CAD build for the part. Positions are in the model's coordinates, mm. A direction names the side the tool comes from. Coordinates: 2 decimals unless noted, no trailing zeros. Loops run counter-clockwise (first coordinate to the right, second up) from the corner with the lowest first, then second, coordinate; pieces in that order, holes last. Notation, with made-up numbers: (82, 8) -> (114, 8) arc R19 ccw to (114, 44) -> close; hole circle Ø1 at (75, 50). An arc over 180 degrees is marked (long way). Write each question's results on one line, items separated by ' | '.
Autodesk Inventor part; units mm, degrees
ref_plane "YZ Plane" through (0, 0, 0) normal (1, 0, 0) x (0, 1, 0)
ref_plane "XZ Plane" through (0, 0, 0) normal (0, 1, 0) x (-1, 0, 0)
ref_plane "XY Plane" through (0, 0, 0) normal (0, 0, 1) x (1, 0, 0)
sketch "Sketch1" plane through (0, 0, 0) normal (0, 1, 0) x (-1, 0, 0)
  line L0 (0.8453, 25) -> (0.8453, 15)
  line L1 (0.8453, 15) -> (4.8453, 15)
  line L2 (4.8453, 15) -> (4.8453, 2)
  line L3 (0.8453, 25) -> (25.8453, 25)
  line L4 (25.8453, 25) -> (25.8453, 6)
  line L5 (4.8453, 2) -> (11.8453, 2)
  line L6 (11.8453, 2) -> (14.1547, 6)
  line L7 (14.1547, 6) -> (25.8453, 6)
  point P0 (0, 0)
  dimension "d1" = 10
  dimension "d2" = 4
  dimension "d3" = 13
  dimension "d13" = 25
  dimension "d14" = 19
  dimension "d16" = 7
  dimension "d17" = 60
  dimension "d19" = 4
revolve "Revolution1" add sketch "Sketch1" angle 360 about axis through (-0.8453, 0, 25) along (-1, 0, 0)
sketch "Sketch2" plane through (-25.8453, 0, 25) normal (-1, 0, 0) x (0, 0, 1)
  circle A0 centre (0, 0) radius 13
  point P0 (-25, 0)
  dimension "d21" = 26
extrude "Extrusion1" cut sketch "Sketch2" against normal blind 15
thread "Thread1"
properties part number "00.32.012 \"Valve\"" material "Steel"
1) Two-plate mould, pull along Y, no slides. Class faces 4 (the flat face through (-10.845, 0, 25)), 5 (the cylindrical face through (-8.394, -22.804, 27.994)), 6 (the flat face through (-25.845, 12.4, 29.5)): pulls with the +Y half, pulls with the -Y half, needs draft (parallel to the pull), parting line crosses it, or undercut.
Outcome:
face 4: undercut | face 5: parting line crosses it | face 6: needs draft
2) Slice it at D-D (x = -8.25). Write the cut outline in (y, z).
Outcome:
outline: circle Ø46 at (0, 25)
3) Drill centre lines: L1, parallel to Y at x = -17.5, z = 25; L2, parallel to X at y = -16.5, z = 28.5; L3, parallel to Z at x = -20.75, y = 8.5. Where is each one in solid material? Low to high. Write a range as from..to.
Outcome:
L1: y = -19..-13, 13..19 | L2: x = -25.85..-4.85 | L3: z = 8.01..15.16, 34.84..41.99
4) Slice it at C-C (x = -20.75). Write the cut outline in (y, z), then the cut area to 3 significant figures.
Outcome:
outline: circle Ø38 at (0, 25); hole circle Ø26 at (0, 25) | area: 603 mm^2
5) Which spindle directions (+Z, -Z, +X, -X, +Y, -Y) get a long thin tool onto all of the face, cutting with end or side? Do faces 1 (the flat face through (-4.845, 5, 15)), 2 (the flat face through (-0.845, 0, 25)), 3 (the cylindrical face through (-18.5, 3.9, 37.4)). Say none if no direction does.
Outcome:
face 1: +X | face 2: +Z, -Z, +X, +Y, -Y | face 3: -X
6) Pin check, flat tips, straight feed: pin 1 (1 mm diameter, centred on y = -17.5, z = 36, fed in from -X); pin 2 (1.5 mm diameter, centred on x = -8.5, y = -18, fed in from +Z); pin 3 (8 mm diameter, centred on y = 13, z = 34, fed in from +X). Stop position of each tip, or through.
Outcome:
pin 1: stops at x = -13.48 | pin 2: stops at z = 40.21 | pin 3: stops at x = -4.85
7) Slice it at A-A (z = 25). Write the cut outline in (x, y), then the cut area to 3 significant figures.
Outcome:
outline: (-25.85, -19) -> (-14.15, -19) -> (-11.85, -23) -> (-4.85, -23) -> (-4.85, -10) -> (-0.85, -10) -> (-0.85, 10) -> (-4.85, 10) -> (-4.85, 23) -> (-11.85, 23) -> (-14.15, 19) -> (-25.85, 19) -> (-25.85, 13) -> (-10.85, 13) -> (-10.85, -13) -> (-25.85, -13) -> close | area: 553 mm^2
8) Slice it at B-B (y = 0). Write the cut outline in (x, z), then the cut area to 3 significant figures.
Outcome:
outline: (-25.85, 6) -> (-14.15, 6) -> (-11.85, 2) -> (-4.85, 2) -> (-4.85, 15) -> (-0.85, 15) -> (-0.85, 35) -> (-4.85, 35) -> (-4.85, 48) -> (-11.85, 48) -> (-14.15, 44) -> (-25.85, 44) -> (-25.85, 38) -> (-10.85, 38) -> (-10.85, 12) -> (-25.85, 12) -> close | area: 553 mm^2
